Answer from the drawing. Dimensions are ordinates in mm from the lowest x, y and z of the part. A direction names the side the tool comes from. Give positions to 0.01 mm unless a question says otherwise; leave off trailing zeros. Loops run counter-clockwise (first coordinate to the right, second up) from the corner with the lowest first, then second, coordinate; pieces in that order, holes last. Notation, with made-up numbers: (70.5, -11) - (78.5, -11) arc R34 ccw to (78.5, 28) - close; hole circle Ø5 at (0, 42.5). An arc over 180 degrees is marked (long way). One line per item, written item: value.
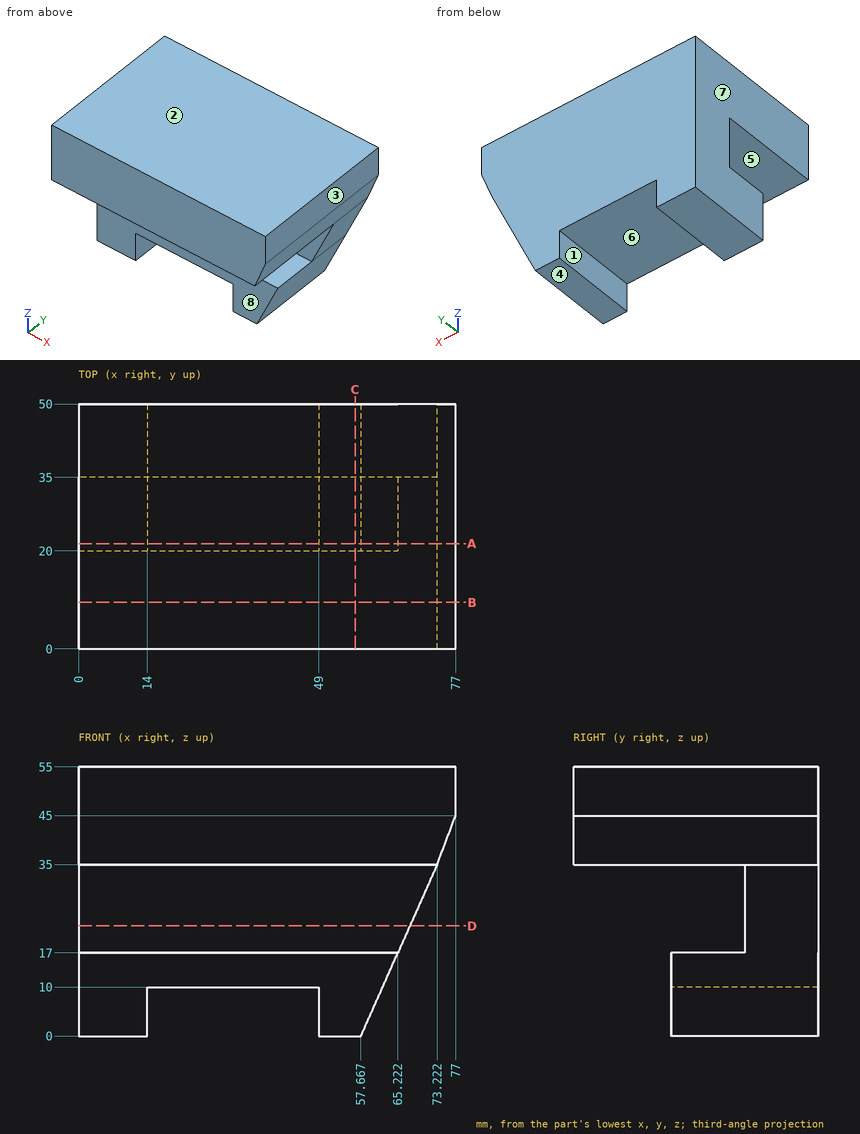
1. Section B-B (y = 9.5) is taken. Write down the section's boundary in (x, z), and give its area (3 significant figures).
Output:
outline: (0, 35) - (73.22, 35) - (77, 45) - (77, 55) - (0, 55) - close
area: 1,520 mm²
2. The mould has two halves that part along X. Classify the marked faces 1, 2 and 3: released by +X, released by -X, zero draft, split by the parting line, or undercut.
Output:
face 1: undercut
face 2: zero draft
face 3: released by +X
3. Section A-A (y = 21.5) is taken. Write down the section's boundary in (x, z).
Output:
outline: (0, 0) - (14, 0) - (14, 10) - (49, 10) - (49, 0) - (57.67, 0) - (65.22, 17) - (0, 17) - close; (0, 35) - (73.22, 35) - (77, 45) - (77, 55) - (0, 55) - close
4. Find the intervals of material crossed by line 1 along Z through (x, y) = (18.5, 3.5); line 2 along X through (y, z) = (44.5, 7.5); line 3 along Y through (x, z) = (7.5, 17.5), in increasing order.
Output:
line 1: z = 35 to 55
line 2: x = 0 to 14, 49 to 61
line 3: y = 35 to 50
5. Section C-C (x = 56.5) is taken. Write down the section's boundary in (y, z), and give its area (3 significant figures).
Output:
outline: (0, 35) - (35, 35) - (35, 17) - (20, 17) - (20, 0) - (50, 0) - (50, 55) - (0, 55) - close
area: 1,780 mm²
6. Section D-D (z = 22.5) is taken. Write down the section's boundary in (x, y), and give its area (4 significant figures).
Output:
outline: (0, 35) - (67.67, 35) - (67.67, 50) - (0, 50) - close
area: 1,015 mm²
7. For the marked faces 4, 5, 6, 7 and 8, determine the directions among +Z, -Z, +X, -X, +Y, -Y from which every point of the face is accessible in a straight line to the end or side of a thin tool.
Output:
face 4: -Z, +X, -X, +Y, -Y
face 5: +X, -X, -Y
face 6: -Z, +Y, -Y
face 7: +Z, -Z, -X, +Y, -Y
face 8: -Z, +X, -X, -Y
8. Flat-ended cylindrical pins translate along their axes: pin 1 Ø5.5 at (x, z) = (25.5, 29.5) entering from -Y; pin 2 Ø5 at (x, z) = (37, 12) entering from -Y; pin 3 Ø1 at (x, z) = (60.5, 38) entering from -Y; pin 4 Ø12 at (x, y) = (16, 9) entering from -Z. Find the tip coordinate at first contact, or state that the pin passes through.
Output:
pin 1: stops at y = 35
pin 2: stops at y = 20
pin 3: stops at y = 0
pin 4: stops at z = 35
